Geometry: see drawing. Coordinates: mm, zero at the bounding-box minimum. A direction names the side the tool comes from. Give positions to 0.01 mm unless a question says otherwise; leave off trailing zeros. Order: outer loops, then holes, each group sorted by start corner. A loop starts at its lowest first (then second) coordinate and runs counter-clockwise, first axis right, second up. Notation, with made-up numbers: M 11.25,55 L 49.25,55 A13 ccw 49.25,74 Z; hole C 8,61.25 d8. An arc over 180 degrees is marked long. Return JSON: item names as keys, results as strings.
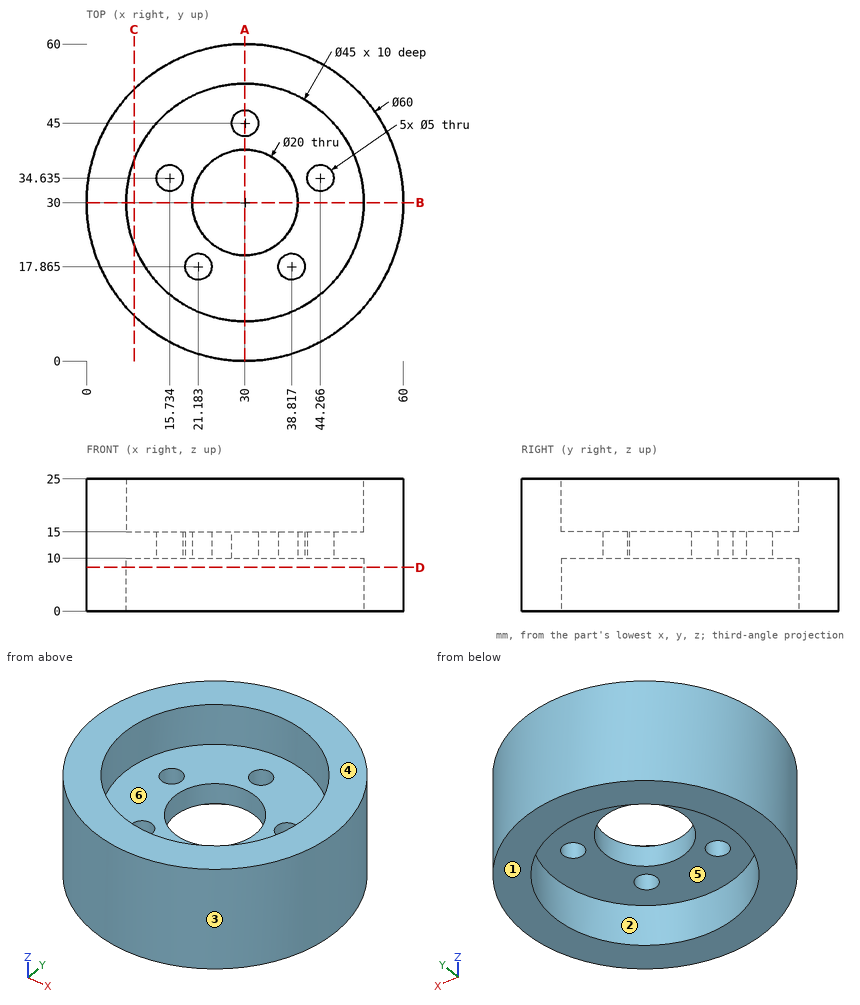
1. Ray query, probe 1 along X at (y, z) = (16, 13); probe 2 along Z at (x, y) = (46.5, 43.5); probe 3 along Y at (x, z) = (15, 12.5) (1 decimal). Return the intervals inside material, ascending.
Evaluation:
{"probe 1": "x = 3.47 to 19.52, 22.85 to 37.15, 40.48 to 56.53", "probe 2": "z = 10 to 15", "probe 3": "y = 4 to 32.2, 37 to 56"}
2. Set-up query: the marked faces 4, 5 and 6. Return all of +Z, -Z, +X, -X, +Y, -Y with unobstructed straight access to the full face (end or side cutting, diameter ignored); none if empty.
Evaluation:
{"face 4": "+Z, +X, -X, +Y, -Y", "face 5": "-Z", "face 6": "+Z"}
3. Section query B-B (y = 30). Return loops of the section in (x, z), then the cut area to 3 significant figures.
Evaluation:
{"outline": "M 0,0 L 7.5,0 L 7.5,10 L 20,10 L 20,15 L 7.5,15 L 7.5,25 L 0,25 Z; M 40,10 L 52.5,10 L 52.5,0 L 60,0 L 60,25 L 52.5,25 L 52.5,15 L 40,15 Z", "area": "500 mm^2"}
4. Draft query along Y for the marked faces 1, 2 and 3. Return one class per face: pulls with the +Y half, pulls with the -Y half, needs draft (parallel to the pull), parting line crosses it, or undercut.
Evaluation:
{"face 1": "needs draft", "face 2": "undercut", "face 3": "parting line crosses it"}
5. Section query A-A (x = 30). Return loops of the section in (y, z), then the cut area to 3 significant figures.
Evaluation:
{"outline": "M 0,0 L 7.5,0 L 7.5,10 L 20,10 L 20,15 L 7.5,15 L 7.5,25 L 0,25 Z; M 40,10 L 42.5,10 L 42.5,15 L 40,15 Z; M 47.5,10 L 52.5,10 L 52.5,0 L 60,0 L 60,25 L 52.5,25 L 52.5,15 L 47.5,15 Z", "area": "475 mm^2"}
6. First-contact query: pin 1 (23 mm diameter, centred on x = 30, y = 30, fed in from +Z); pin 2 (8 mm diameter, centred on x = 44, z = 7, fed in from +Y); pin 3 (1 mm diameter, centred on x = 43.5, z = 15, fed in from -Y); pin 4 (5 mm diameter, centred on x = 23.5, y = 29, fed in from +Z). Flat tips, straight axial feed; report the tip coordinate or a pass-through.
Evaluation:
{"pin 1": "stops at z = 15", "pin 2": "stops at y = 58.28", "pin 3": "stops at y = 2.96", "pin 4": "passes through"}
7. Section query D-D (z = 8.25). Return loops of the section in (x, y).
Evaluation:
{"outline": "C 30,30 d60; hole C 30,30 d45"}
8. Section query C-C (x = 9). Return loops of the section in (y, z).
Evaluation:
{"outline": "M 8.58,0 L 21.92,0 L 21.92,10 L 38.08,10 L 38.08,0 L 51.42,0 L 51.42,25 L 38.08,25 L 38.08,15 L 21.92,15 L 21.92,25 L 8.58,25 Z"}
